```python
from build123d import *

# Parameters (mm, degrees)
F0_W     = 400
F0_H     = 120
F0_R     = 12.7
F0_R_2   = 6.35
F1_DEPTH = 60
F3_D     = 12
F3_DEPTH = 80
F3_TIP   = 3.6051637142
F4_D     = 12.7


with BuildPart() as f1:
    # F0 (on Top) → F1 (new body)
    with BuildSketch(Plane.XY):
        with Locations((0, 60)):
            Rectangle(F0_W, F0_H)
        with Locations((-80, 20)):
            Circle(F0_R, mode=Mode.SUBTRACT)
        with Locations((0, 20)):
            Circle(F0_R, mode=Mode.SUBTRACT)
        with Locations((80, 20)):
            Circle(F0_R, mode=Mode.SUBTRACT)
        with Locations((160, 20)):
            Circle(F0_R, mode=Mode.SUBTRACT)
        with Locations((-160, 100)):
            Circle(F0_R, mode=Mode.SUBTRACT)
        with Locations((-80, 100)):
            Circle(F0_R, mode=Mode.SUBTRACT)
        with Locations((0, 100)):
            Circle(F0_R, mode=Mode.SUBTRACT)
        with Locations((80, 100)):
            Circle(F0_R, mode=Mode.SUBTRACT)
        with Locations((160, 100)):
            Circle(F0_R, mode=Mode.SUBTRACT)
        with Locations((-160, 100)):
            Circle(F0_R)
        with Locations((-160, 100)):
            Circle(F0_R_2, mode=Mode.SUBTRACT)
        with Locations((-80, 100)):
            Circle(F0_R)
        with Locations((-80, 100)):
            Circle(F0_R_2, mode=Mode.SUBTRACT)
        with Locations((0, 100)):
            Circle(F0_R)
        with Locations((0, 100)):
            Circle(F0_R_2, mode=Mode.SUBTRACT)
        with Locations((80, 100)):
            Circle(F0_R)
        with Locations((80, 100)):
            Circle(F0_R_2, mode=Mode.SUBTRACT)
        with Locations((160, 100)):
            Circle(F0_R)
        with Locations((160, 100)):
            Circle(F0_R_2, mode=Mode.SUBTRACT)
        with Locations((80, 20)):
            Circle(F0_R)
        with Locations((80, 20)):
            Circle(F0_R_2, mode=Mode.SUBTRACT)
        with Locations((160, 20)):
            Circle(F0_R)
        with Locations((160, 20)):
            Circle(F0_R_2, mode=Mode.SUBTRACT)
        with Locations((0, 20)):
            Circle(F0_R)
        with Locations((0, 20)):
            Circle(F0_R_2, mode=Mode.SUBTRACT)
        with Locations((-80, 20)):
            Circle(F0_R)
        with Locations((-80, 20)):
            Circle(F0_R_2, mode=Mode.SUBTRACT)
        with Locations((-160, 100)):
            Circle(F0_R_2)
        with Locations((-80, 100)):
            Circle(F0_R_2)
        with Locations((0, 100)):
            Circle(F0_R_2)
        with Locations((80, 100)):
            Circle(F0_R_2)
        with Locations((160, 100)):
            Circle(F0_R_2)
        with Locations((80, 20)):
            Circle(F0_R_2)
        with Locations((160, 20)):
            Circle(F0_R_2)
        with Locations((0, 20)):
            Circle(F0_R_2)
        with Locations((-80, 20)):
            Circle(F0_R_2)
    extrude(amount=-F1_DEPTH)

    # F3
    with Locations(Plane.XZ):
        with Locations((-120, -12), (-120, -48), (120, -48), (120, -12)):
            Hole(F3_D / 2, depth=F3_DEPTH)
            with Locations((0, 0, -(F3_DEPTH + F3_TIP / 2))):  # 118° drill point
                Cone(0, F3_D / 2, F3_TIP, mode=Mode.SUBTRACT)

    # F4 (through all)
    with Locations(Plane.XY):
        with Locations((-80, 20), (-80, 100), (-160, 100), (0, 100), (0, 20), (80, 20), (80, 100), (160, 100), (160, 20)):
            Hole(F4_D / 2)


solid = f1.part
```
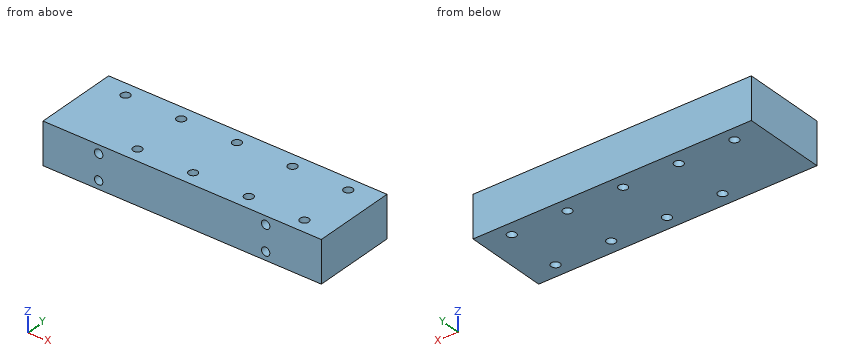
Input: part model. Units: mm. Frame: model coordinates. Round coordinates to 2 decimals unless told otherwise and drop trailing zeros. Order: outer loops, then holes, each group sorted by start corner. A loop starts at its lowest first (then second) coordinate and runs counter-clockwise, first axis right, second up. Notation, with made-up numbers: (84.5, 32) - (111.5, 32) arc R14 ccw to (111.5, 47) - close; hole circle Ø8 at (9, 74.25). An arc over 180 degrees is marked (long way). One line per question, with ' | ' between items. Start each with the question number.
1) Cut plane A-A, the plane x = 80. Return the cut outline in (y, z).
2) Contact query for flat-ended pins moving along their axis: P1, Ø7.5, axis at x = 0, y = 20, coming from the +Z side; P2, Ø9.5, axis at x = 120, z = -48, coming from the -Y side. Output: stop coordinate, or through.
3) Cut plane D-D, the plane y = 74. Return the cut outline in (x, z).
4) Cut plane B-B, the plane y = 100. Return the cut outline in (x, z), then the cut area to 3 significant figures.
5) Ray query, probe 1 along Y at (x, z) = (0, -14.5); probe 2 along X at (y, z) = (44.5, -48); probe 3 along Y at (x, z) = (-160, -19). Return the intervals inside material, ascending.
6) Cut plane C-C, the plane z = -22. Give the number of separate pieces and of enclosed holes in the cut face, then the cut area to 3 significant figures.
Worked out:
1) outline: (0, -60) - (13.65, -60) - (13.65, 0) - (0, 0) - close; (26.35, -60) - (93.65, -60) - (93.65, 0) - (26.35, 0) - close; (106.35, -60) - (120, -60) - (120, 0) - (106.35, 0) - close
2) P1: passes through | P2: stops at y = 80.75
3) outline: (-200, -60) - (200, -60) - (200, 0) - (-200, 0) - close; hole circle Ø12 at (-120, -48); hole circle Ø12 at (-120, -12); hole circle Ø12 at (120, -48); hole circle Ø12 at (120, -12)
4) outline: (-200, -60) - (-166.35, -60) - (-166.35, 0) - (-200, 0) - close; (-153.65, -60) - (-86.35, -60) - (-86.35, 0) - (-153.65, 0) - close; (-73.65, -60) - (-6.35, -60) - (-6.35, 0) - (-73.65, 0) - close; (6.35, -60) - (73.65, -60) - (73.65, 0) - (6.35, 0) - close; (86.35, -60) - (153.65, -60) - (153.65, 0) - (86.35, 0) - close; (166.35, -60) - (200, -60) - (200, 0) - (166.35, 0) - close | area: 20,200 mm^2
5) probe 1: y = 0 to 13.65, 26.35 to 93.65, 106.35 to 120 | probe 2: x = -200 to -126, -114 to 114, 126 to 200 | probe 3: y = 0 to 93.65, 106.35 to 120
6) separate pieces: 1 | enclosed holes: 9 | area: 46,900 mm^2
